```python
from build123d import *

# Parameters (mm, degrees)
SKETCH1_W           = 140
SKETCH1_H           = 140
BOSS_EXTRUDE1_DEPTH = 3.175
SKETCH2_W           = 30
SKETCH2_H           = 30
BOSS_EXTRUDE2_DEPTH = 10
SKETCH11_W          = 30
SKETCH11_H          = 10
BOSS_EXTRUDE3_DEPTH = 10
SKETCH13_W          = 30
SKETCH13_H          = 10
BOSS_EXTRUDE4_DEPTH = 10
SKETCH16_W          = 30
SKETCH16_H          = 10
BOSS_EXTRUDE6_DEPTH = 10
SKETCH17_W          = 30
SKETCH17_H          = 10
BOSS_EXTRUDE7_DEPTH = 10
SKETCH18_R          = 6.05
CUT_EXTRUDE1_DEPTH  = 13.175
SKETCH21_R          = 1.65
CUT_EXTRUDE2_DEPTH  = 3.175
SKETCH22_R          = 2.05
CUT_EXTRUDE3_DEPTH  = 1


with BuildPart() as part:
    # Sketch1 → Boss-Extrude1 (new body)
    with BuildSketch(Plane(origin=(0, 0, 0), x_dir=(1, 0, 0), z_dir=(0, 1, 0))):
        Rectangle(SKETCH1_W, SKETCH1_H)
    extrude(amount=BOSS_EXTRUDE1_DEPTH)

    # Sketch2 → Boss-Extrude2 (add)
    with BuildSketch(Plane(origin=(0, 3.175, 0), x_dir=(1, 0, 0), z_dir=(0, 1, 0))):
        with Locations((45, -45.5)):
            Rectangle(SKETCH2_W, SKETCH2_H)
        with Locations((-45, -45.5)):
            Rectangle(SKETCH2_W, SKETCH2_H)
        with Locations((-45, 45.5)):
            Rectangle(SKETCH2_W, SKETCH2_H)
    boss_extrude2 = extrude(amount=BOSS_EXTRUDE2_DEPTH)

    # Sketch11 → Boss-Extrude3 (add)
    with BuildSketch(Plane.ZY.offset(60)):
        with Locations((45.5, 8.175)):
            Rectangle(SKETCH11_W, SKETCH11_H)
    extrude(amount=BOSS_EXTRUDE3_DEPTH)

    # Sketch13 → Boss-Extrude4 (add)
    with BuildSketch(Plane(origin=(60, 0, 0), x_dir=(0, 0, -1), z_dir=(1, 0, 0))):
        with Locations((-45.5, 8.175)):
            Rectangle(SKETCH13_W, SKETCH13_H)
    extrude(amount=BOSS_EXTRUDE4_DEPTH)

    # Mirror1: Boss-Extrude2 across plane
    add(boss_extrude2.mirror(Plane(origin=(0, 0, 0), x_dir=(0, 0, 1), z_dir=(1, 0, 0))))

    # Sketch16 → Boss-Extrude6 (add)
    with BuildSketch(Plane(origin=(60, 0, 0), x_dir=(0, 0, -1), z_dir=(1, 0, 0))):
        with Locations((45.5, 8.175)):
            Rectangle(SKETCH16_W, SKETCH16_H)
    extrude(amount=BOSS_EXTRUDE6_DEPTH)

    # Sketch17 → Boss-Extrude7 (add)
    with BuildSketch(Plane.ZY.offset(60)):
        with Locations((-45.5, 8.175)):
            Rectangle(SKETCH17_W, SKETCH17_H)
    extrude(amount=BOSS_EXTRUDE7_DEPTH)

    # Sketch18 → Cut-Extrude1 (cut)
    with BuildSketch(Plane(origin=(0, 13.175, 0), x_dir=(1, 0, 0), z_dir=(0, 1, 0))):
        with Locations(Location((-57.9286, -45.5, 0), (0, 0, 270))):
            Circle(SKETCH18_R)
        with Locations(Location((57.9286, -45.5, 0), (0, 0, 90))):
            Circle(SKETCH18_R)
    extrude(amount=-CUT_EXTRUDE1_DEPTH, mode=Mode.SUBTRACT)

    # Sketch21 → Cut-Extrude2 (cut)
    with BuildSketch(Plane(origin=(0, 0, 0), x_dir=(-1, 0, 0), z_dir=(0, -1, 0))):
        with Locations(Location((-62.9286, -11, 0), (0, 0, 90))):
            Circle(SKETCH21_R)
        with Locations(Location((-52.9286, -11, 0), (0, 0, 90))):
            Circle(SKETCH21_R)
        with Locations(Location((-62.9286, -60, 0), (0, 0, 90))):
            Circle(SKETCH21_R)
        with Locations(Location((-52.9286, -60, 0), (0, 0, 90))):
            Circle(SKETCH21_R)
        with Locations(Location((52.9286, -11, 0), (0, 0, 90))):
            Circle(SKETCH21_R)
        with Locations(Location((62.9286, -11, 0), (0, 0, 90))):
            Circle(SKETCH21_R)
        with Locations(Location((52.9286, -60, 0), (0, 0, 90))):
            Circle(SKETCH21_R)
        with Locations(Location((62.9286, -60, 0), (0, 0, 90))):
            Circle(SKETCH21_R)
    extrude(amount=-CUT_EXTRUDE2_DEPTH, mode=Mode.SUBTRACT)

    # Sketch22 → Cut-Extrude3 (cut)
    with BuildSketch(Plane(origin=(0, 3.175, 0), x_dir=(-1, 0, 0), z_dir=(0, -1, 0))):
        with Locations((62.9286, -60)):
            Circle(SKETCH22_R)
        with Locations((52.9286, -60)):
            Circle(SKETCH22_R)
        with Locations((-52.9286, -60)):
            Circle(SKETCH22_R)
        with Locations((-62.9286, -60)):
            Circle(SKETCH22_R)
    extrude(amount=-CUT_EXTRUDE3_DEPTH, mode=Mode.SUBTRACT)


solid = part.part
```
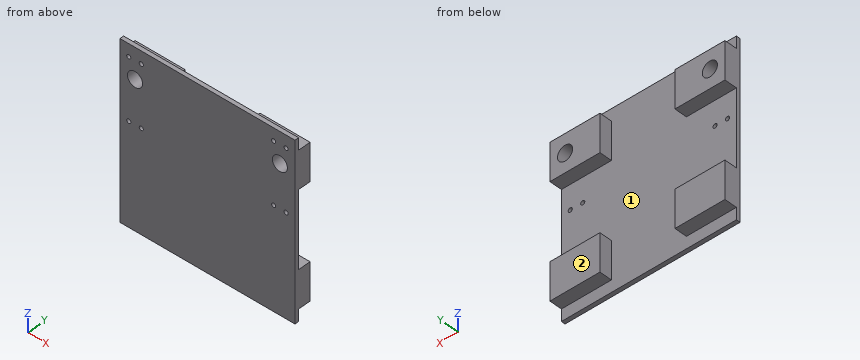
Part model, mm, in its own coordinate system. Face numbers are marked on the shaded views. Coordinates: 2 decimals unless noted, no trailing zeros. Order: outer loops, then holes, each group sorted by start corner. A loop starts at its lowest first (then second) coordinate and runs counter-clockwise, first axis right, second up. Notation, with made-up numbers: (84, 78) - (102, 78) arc R13 cw to (102, 96) - close; hole circle Ø8 at (36, -10.75). An arc over 180 degrees is marked (long way). Return JSON: item names as keys, results as strings. Group by question number.
Item 1: Cut at C-C (y = 9). List the corners of the cut face in (x, z).
Item 2: Drill centre lines: probe 1 along X at (y, z) = (2.45, 11); probe 2 along X at (y, z) = (3.8, 60); probe 3 along Z at (x, y) = (-34.5, 4). Where is each one in solid material? Low to high. Write a range as from..to.
Item 3: Cut at A-A (z = 11). List the corners of the cut face in (x, y) (3 decimals), plus the area to 3 significant figures.
Item 4: Cut at D-D (x = -42.5). List the corners of the cut face in (y, z) (3 decimals).
Item 5: Pin check, flat tips, straight feed: pin 1 (2 mm diameter, centred on x = -52.93, z = 11, fed in from -Y); pin 2 (3 mm diameter, centred on x = 52, y = 8.5, fed in from +Z); pin 3 (4 mm diameter, centred on x = -25.5, z = -12.5, fed in from +Y) (3 decimals). Stop position of each tip, or through.
Item 6: Pull direction X, two halves, no side cores. Call the marked faces 1 and 2: pulls with the +X half, pulls with the -X half, needs draft (parallel to the pull), parting line crosses it, or undercut.
Item 7: Cut at B-B (z = 45.5). List the corners of the cut face in (x, y) (3 decimals), plus the area to 3 significant figures.
Check values:
{
 "1": {"outline": "(-70, -60.5) - (-30, -60.5) - (-30, -30.5) - (-70, -30.5) - close; (-70, 30.5) - (-30, 30.5) - (-30, 60.5) - (-70, 60.5) - close; (30, -60.5) - (70, -60.5) - (70, -30.5) - (30, -30.5) - close; (30, 30.5) - (70, 30.5) - (70, 60.5) - (30, 60.5) - close; hole circle Ø12.1 at (-57.93, 45.5); hole circle Ø12.1 at (57.93, 45.5)"},
 "2": {"probe 1": "x = -70..-64.58, -61.28..-54.58, -51.28..51.28, 54.58..61.28, 64.58..70", "probe 2": "x = -70..-64.98, -60.88..-54.98, -50.88..-30, 30..50.88, 54.98..60.88, 64.98..70", "probe 3": "z = -60.5..-30.5, 30.5..60.5"},
 "3": {"outline": "(-70, 0) - (-64.579, 0) - (-64.579, 3.175) - (-70, 3.175) - close; (-61.279, 0) - (-54.579, 0) - (-54.579, 3.175) - (-61.279, 3.175) - close; (-51.279, 0) - (51.279, 0) - (51.279, 3.175) - (-51.279, 3.175) - close; (54.579, 0) - (61.279, 0) - (61.279, 3.175) - (54.579, 3.175) - close; (64.579, 0) - (70, 0) - (70, 3.175) - (64.579, 3.175) - close", "area": "403 mm2"},
 "4": {"outline": "(0, -70) - (3.175, -70) - (3.175, -60.5) - (13.175, -60.5) - (13.175, -30.5) - (3.175, -30.5) - (3.175, 30.5) - (13.175, 30.5) - (13.175, 60.5) - (3.175, 60.5) - (3.175, 70) - (0, 70) - close"},
 "5": {"pin 1": "passes through", "pin 2": "stops at z = 60.5", "pin 3": "stops at y = 3.175"},
 "6": {"face 1": "undercut", "face 2": "needs draft"},
 "7": {"outline": "(-70, 0) - (-63.979, 0) - (-63.979, 13.175) - (-70, 13.175) - close; (-51.879, 0) - (51.879, 0) - (51.879, 13.175) - (30, 13.175) - (30, 3.175) - (-30, 3.175) - (-30, 13.175) - (-51.879, 13.175) - close; (63.979, 0) - (70, 0) - (70, 13.175) - (63.979, 13.175) - close", "area": "926 mm2"}
}
